```python
from build123d import *

# Parameters (mm, degrees)
CUT_EXTRUDE1_DEPTH = 2.5


with BuildPart() as part:
    # Sketch1 → Revolve1 (revolve)
    with BuildSketch(Plane(origin=(0, 0, 0), x_dir=(1, 0, 0), z_dir=(0, 1, 0))):
        Polygon((0, 0), (12.5, 0), (12.5, 4), (10, 4.5), (0, 4.5), align=None)
    revolve(axis=Axis((0, 0, 0), (1, 0, 0)))

    # Sketch2 → Cut-Extrude1 (cut)
    with BuildSketch(Plane(origin=(12.5, 0, 0), x_dir=(0, 0, -1), z_dir=(1, 0, 0))):
        with BuildLine():
            Line((-2, -4.031128874), (-2, 4.031128874))
            ThreePointArc((-2, 4.031128874), (-4.5, 0), (-2, -4.031128874))
        make_face()
        with BuildLine():
            Line((2, -4.031128874), (2, 4.031128874))
            ThreePointArc((2, 4.031128874), (4.5, 0), (2, -4.031128874))
        make_face()
    extrude(amount=-CUT_EXTRUDE1_DEPTH, mode=Mode.SUBTRACT)


solid = part.part
```
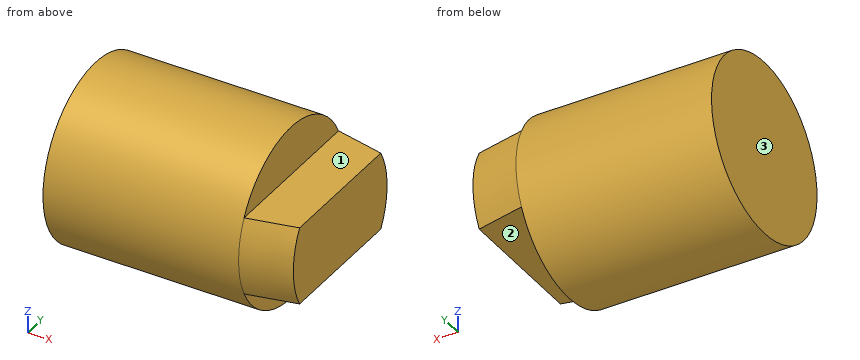
Geometry check sheet. Reference: the model listing, model coordinates, mm. Face numbers are marked on the shaded views. A direction names the side the tool comes from. Coordinates: 2 decimals unless noted, no trailing zeros. Order: outer loops, then holes, each group sorted by start corner. A loop starts at its lowest first (then second) coordinate and runs counter-clockwise, first axis right, second up.
Item 1: Scan lines: line 1 along X through (y, z) = (-0.5, -3.75); line 2 along Z through (x, y) = (2, 2); line 3 along Z through (x, y) = (12, 3.25). Record each from-to range of solid material in increasing order.
Item 2: Depth check by flat-ended pin: pin 1 (0.8 mm diameter, centred on x = 11.5, y = -0.5, fed in from +Z); pin 2 (3 mm diameter, centred on y = -1, z = 4, fed in from +X); pin 3 (1.3 mm diameter, centred on x = 12, y = -0.5, fed in from -Z). Enter the tip coordinate at first touch or a pass-through.
Item 3: Section check B-B (x = 2.5). Enter the section's corners in (y, z).
Item 4: Tool access check on the marked faces 1, 2 and 3. Record the directions out of +Z, -Z, +X, -X, +Y, -Y that give a thin tool (end or side, any length) a straight path to the whole face; none if there is none.
Item 5: Section check C-C (y = 3). Enter the section's corners in (x, z).
Item 6: Section check D-D (x = 10.75). Enter the section's corners in (y, z), plus the area to 3 significant figures.
Item 7: Section check A-A (y = 0). Enter the section's corners in (x, z).
Check sheet entries:
1. line 1: x = 0 to 10
1. line 2: z = -4.03 to 4.03
1. line 3: z = -2 to 2
2. pin 1: stops at z = 2
2. pin 2: stops at x = 10
2. pin 3: stops at z = -2
3. outline: circle Ø9 at (0, 0)
4. face 1: +Z, +X, +Y, -Y
4. face 2: -Z, +X, +Y, -Y
4. face 3: +Z, -Z, -X, +Y, -Y
5. outline: (0, -3.35) - (10, -3.35) - (10, -2) - (12.5, -2) - (12.5, 2) - (10, 2) - (10, 3.35) - (0, 3.35) - close
6. outline: (-3.86, -2) - (3.86, -2) arc R4.35 ccw to (3.86, 2) - (-3.86, 2) arc R4.35 ccw to start
6. area: 33.5 mm2
7. outline: (0, -4.5) - (10, -4.5) - (10, -2) - (12.5, -2) - (12.5, 2) - (10, 2) - (10, 4.5) - (0, 4.5) - close
